```python
from build123d import *

# Parameters (mm, degrees)
F1_DEPTH = 136.652
F2_DEPTH = 136.653
F0_W     = 124.218264
F0_H     = 78.966799
F0_W_2   = 121.818223
F3_DEPTH = 136.653


with BuildPart() as f1:
    # F0 (on Front) → F1 (new body)
    with BuildSketch(Plane.XZ):
        with BuildLine():
            Line((68.681777, -30.518653), (68.681777, 48.448146))
            Line((68.681777, 48.448146), (50.39659, 48.448146))
            ThreePointArc((50.39659, 48.448146), (0, -12.265111), (-50.39659, 48.448146))
            Line((-50.39659, 48.448146), (-66.281736, 48.448146))
            Line((-66.281736, 48.448146), (-66.281736, -30.518653))
            Line((-66.281736, -30.518653), (-190.5, -30.518653))
            Line((-190.5, -30.518653), (-190.5, -48.448146))
            Line((-190.5, -48.448146), (190.5, -48.448146))
            Line((190.5, -48.448146), (190.5, -30.518653))
            Line((190.5, -30.518653), (68.681777, -30.518653))
        make_face()
        with BuildLine():
            ThreePointArc((-50.39659, 48.448146), (0, -12.265111), (50.39659, 48.448146))
            Line((50.39659, 48.448146), (-50.39659, 48.448146))
        make_face()
    extrude(amount=-F1_DEPTH)

    # F0 (on Front) → F2 (cut, through all)
    with BuildSketch(Plane.XZ):
        with BuildLine():
            ThreePointArc((-50.39659, 48.448146), (0, -12.265111), (50.39659, 48.448146))
            Line((50.39659, 48.448146), (-50.39659, 48.448146))
        make_face()
    extrude(amount=-F2_DEPTH, mode=Mode.SUBTRACT)

    # F0 (on Front) → F3 (cut, through all)
    with BuildSketch(Plane.XZ):
        with Locations((-128.390868, 8.964747)):
            Rectangle(F0_W, F0_H)
        with Locations((129.590889, 8.964747)):
            Rectangle(F0_W_2, F0_H)
    extrude(amount=-F3_DEPTH, mode=Mode.SUBTRACT)


solid = f1.part
```
Model file for the job. Use its own axes, mm. A direction names the side the tool comes from. Round coordinates to 2 decimals unless told otherwise and drop trailing zeros. Write each loop counter-clockwise with the first axis right and the second up, starting at its lowest first coordinate (ties: lowest second). Pieces come first, ordered by that corner, then holes. Notation, with made-up numbers: (25, -3) -> (40, -3) arc R13 ccw to (40, 12) -> close; hole circle Ø2 at (7, 10.5). An arc over 180 degrees is marked (long way). Answer as CSV lines item,"result".
1. Drill centre lines: line 1 (Z direction, x = 123.5, y = 131); line 2 (Z direction, x = 0, y = 28); line 3 (X direction, y = 109.5, z = -27.5). Where is each one in solid material? Low to high.
Resolved:
line 1,"-48.45 to -30.52"
line 2,"-48.45 to -12.27"
line 3,"-66.28 to 68.68"
2. Slice it at D-D, the plane z = -16. List the corners of the cut face in (x, y).
Resolved:
outline,"(-66.28, 0) -> (68.68, 0) -> (68.68, 136.65) -> (-66.28, 136.65) -> close"
3. Slice it at C-C, the plane x = -101. List the corners of the cut face in (y, z), plus the area to 3 significant figures.
Resolved:
outline,"(0, -48.45) -> (136.65, -48.45) -> (136.65, -30.52) -> (0, -30.52) -> close"
area,"2,450 mm²"
4. Slice it at A-A, the plane z = 22. List the corners of the cut face in (x, y), plus the area to 3 significant figures.
Resolved:
outline,"(-66.28, 0) -> (-48.37, 0) -> (-48.37, 136.65) -> (-66.28, 136.65) -> close; (48.37, 0) -> (68.68, 0) -> (68.68, 136.65) -> (48.37, 136.65) -> close"
area,"5,220 mm²"
5. Tool access for faces 5 (the face through (190.5, 67, -40)), 6 (the face through (130, 67, -30.519)): list every direction of +Z, -Z, +X, -X, +Y, -Y with a clear straight run to the whole face (end or side of a thin tool).
Resolved:
face 5,"+Z, -Z, +X, +Y, -Y"
face 6,"+Z, +X, +Y, -Y"
6. Pin check, flat tips, straight feed: pin 1 Ø6 at (x, y) = (14, 95) entering from +Z; pin 2 Ø23.5 at (y, z) = (86.5, 10) entering from -X; pin 3 Ø10 at (x, y) = (78, 45) entering from +Z. Stop position of each tip, or through.
Resolved:
pin 1,"z = -9.36"
pin 2,"x = -66.28"
pin 3,"z = -30.52"
7. Mould opens along Z. For faces 1 (the face through (-3, 67, -48.448)), 2 (the face through (-128, 67, -30.519)), 3 (the face through (-1.26, 67.37, -12.25)), 4 (the face through (-66.282, 67, 10)) say: +Z half, -Z half, draft (parallel to the pull), parting line (faces both ways), or undercut.
Resolved:
face 1,"-Z half"
face 2,"+Z half"
face 3,"undercut"
face 4,"draft"
8. Slice it at B-B, the plane y = 54.5. List the corners of the cut face in (x, z), plus the area to 3 significant figures.
Resolved:
outline,"(-190.5, -48.45) -> (190.5, -48.45) -> (190.5, -30.52) -> (68.68, -30.52) -> (68.68, 48.45) -> (50.4, 48.45) arc R51.27 cw (long way) to (-50.4, 48.45) -> (-66.28, 48.45) -> (-66.28, -30.52) -> (-190.5, -30.52) -> close"
area,"12,400 mm²"
